Design review of the part built by this model. Coordinates are the model's own, in mm. A direction names the side the tool comes from. Coordinates: 2 decimals unless noted, no trailing zeros. Write each loop counter-clockwise with the first axis right and the second up, starting at its lowest first coordinate (ties: lowest second). Pieces come first, ordered by that corner, then holes.
Q1. Machinability: for faces 1 (the face through (0, 24, 1.7)), 2 (the face through (0, 37, 3.2)), 3 (the face through (0, 16, 4.9)), which of the approach directions +Z, -Z, +X, -X, +Y, -Y give a long, thin tool a straight path to every point of the face, cutting with its end or side? Answer none if there is none.
Q2. Clearance check with a flat-ended pin moving along its axis: pin 1 Ø1.4 at (x, y) = (0, 15.5) entering from -Z. State where the tip first meets the part, or that it passes through.
Q3. Add section B-B, the plane y = 72. Give the boundary of the cut face in (x, z).
Q4. To check wall thickness, follow probe 1 along Z at (x, y) = (-0.5, 27.5); probe 2 along Z at (x, y) = (1.25, 26); probe 3 along X at (y, z) = (50, 1.45). State the ranges of each line that lie inside material, in increasing order.
Q5. Add section A-A, the plane z = 4.25. Give the number of separate pieces and of enclosed holes in the cut face, plus the area to 3 significant figures.
Autodesk Inventor part; units mm, degrees
ref_plane "YZ Plane" through (0, 0, 0) normal (1, 0, 0) x (0, 1, 0)
ref_plane "XZ Plane" through (0, 0, 0) normal (0, 1, 0) x (-1, 0, 0)
ref_plane "XY Plane" through (0, 0, 0) normal (0, 0, 1) x (1, 0, 0)
sketch "Sketch1" plane through (0, 0, 0) normal (0, 0, 1) x (1, 0, 0)
  line L0 (-4, -4) -> (4, -4)
  line L1 (4, -4) -> (4, 4)
  line L2 (4, 4) -> (-4, 4)
  line L3 (-4, 4) -> (-4, -4)
  line L4 (-4, -4) -> (4, 4) construction
  line L5 (4, -4) -> (-4, 4) construction
  circle A0 centre (0, 0) radius 2.4
  dimension "d0" = 8
  dimension "d1" = 8
  dimension "d2" = 4.8
extrude "Extrusion1" add sketch "Sketch1" along normal blind 3.2 contours L3 L2 L1 L0 | A0
extrude "Extrusion2" add sketch "Sketch1" along normal blind 4.9 contours A0
extrude "Extrusion3" cut sketch "Sketch1" along normal blind 1.7 contours A0
pattern_linear "Rectangular Pattern1" count 10 spacing 8 along (0, 1, 0) of "Extrusion1", "Extrusion2", "Extrusion3"
equation "\"d11\" = d0"
equation "\"d24\" = d0"
properties part number "LEGO Plate 1x10"
Here are the results:
1. face 1: -Z
1. face 2: +Z
1. face 3: +Z, +X, -X, +Y, -Y
2. pin 1: stops at z = 1.7
3. outline: (-4, 0) - (-2.4, 0) - (-2.4, 1.7) - (2.4, 1.7) - (2.4, 0) - (4, 0) - (4, 3.2) - (2.4, 3.2) - (2.4, 4.9) - (-2.4, 4.9) - (-2.4, 3.2) - (-4, 3.2) - close
4. probe 1: z = 0 to 3.2
4. probe 2: z = 1.7 to 4.9
4. probe 3: x = -4 to -1.33, 1.33 to 4
5. separate pieces: 10
5. enclosed holes: 0
5. area: 181 mm2
